The listing builds one solid part. Answer for the finished solid, in the listing's coordinates (mm). Face numbers are marked on the shaded views. A direction names the side the tool comes from. Coordinates: 2 decimals unless noted, no trailing zeros. Loops run counter-clockwise (first coordinate to the right, second up) from the corner with the lowest first, then second, coordinate; pieces in that order, holes last. Notation, with made-up numbers: M 10,2 L 32,2 A27 ccw 32,28 Z; hole C 83,79 d9. An arc over 180 degrees is marked long. Return JSON: item names as keys, results as strings. Group by question number.
1. Which of the six approach directions +Z, -Z, +X, -X, +Y, -Y give full straight-line access (tool end or side, diameter ignored) to the marked faces 1, 2 and 3?
2. Section C-C (y = -13) is taken. Count the separate pieces of the cut face and the enclosed holes in it, then the cut area to 3 significant figures.
3. Section A-A (y = 9.25) is taken. Write down the section's boundary in (x, z), then the cut area to 4 significant figures.
4. Section D-D (y = 3.5) is taken. Write down the section's boundary in (x, z), then the cut area to 3 significant figures.
5. Given P1, Ø4.5, axis at x = 4.5, y = 9.25, coming from the -Z side; P2, Ø8, axis at x = 2.5, y = -20.5, coming from the +Z side; P3, Ø1, axis at x = 2, z = 3, coming from the -Y side; P4, Ø0.6, axis at y = -4.5, z = 0.5, coming from the -X side, each flat-ended and moving along its own axis, determine where each tip first touches the part or whether it passes through.
6. The mould has two halves that part along Y. Classify the marked faces 4, 5 and 6: pulls with the +Y half, pulls with the -Y half, needs draft (parallel to the pull), parting line crosses it, or undercut.
7. Section B-B (y = 17.75) is taken. Write down the section's boundary in (x, z), then the cut area to 4 significant figures.
8. Straight lines are drawn through the part: L1, parallel to Y at x = -11.5, z = 6.75; L2, parallel to X at y = 9.25, z = 1; L3, parallel to X at y = -12, z = 5. For each, find the intervals that lie inside material, in ascending order. Write a range as from..to.
```python
from build123d import *

# Parameters (mm, degrees)
SKETCH_W        = 27.5
SKETCH_H        = 57.5
SKETCH_R        = 1.75
PAD_DEPTH       = 9
POCKET_DEPTH    = 7
SKETCH002_W     = 24.5
SKETCH002_H     = 54.5
POCKET001_DEPTH = 3
SKETCH003_W     = 0.8
SKETCH003_H     = 5
PAD001_DEPTH    = 1.4
CHAMFER_SIZE    = 0.6
SKETCH004_W     = 20
SKETCH004_H     = 3
POCKET002_DEPTH = 9.001
SKETCH005_W     = 22.5
SKETCH005_H     = 2
PAD002_DEPTH    = 2
POCKET003_DEPTH = 2.001
CHAMFER001_SIZE = 2.5


with BuildPart() as part:
    # Sketch → Pad (new body)
    with BuildSketch(Plane.XY):
        Rectangle(SKETCH_W, SKETCH_H)
        with Locations((-4.5, 9.25)):
            Circle(SKETCH_R, mode=Mode.SUBTRACT)
        with Locations((-4.5, -25.75)):
            Circle(SKETCH_R, mode=Mode.SUBTRACT)
        with Locations((4.5, 9.25)):
            Circle(SKETCH_R, mode=Mode.SUBTRACT)
        with Locations((4.5, -25.75)):
            Circle(SKETCH_R, mode=Mode.SUBTRACT)
    extrude(amount=PAD_DEPTH)

    # Sketch001 (on Face10 of Pad) → Pocket (cut)
    with BuildSketch(Plane.XY.offset(9)):
        Polygon((-11.25, 26.25), (11.25, 26.25), (11.25, -26.25), (8, -26.25), (8, -29.25), (-8, -29.25), (-8, -26.25), (-11.25, -26.25), align=None)
    extrude(amount=-POCKET_DEPTH, mode=Mode.SUBTRACT)

    # Sketch002 (on Face5 of Pocket) → Pocket001 (cut)
    with BuildSketch(Plane.XY.offset(9)):
        Rectangle(SKETCH002_W, SKETCH002_H)
    extrude(amount=-POCKET001_DEPTH, mode=Mode.SUBTRACT)

    # Sketch003 (on Face5 of Pocket001) → Pad001 (join)
    with BuildSketch(Plane.XY.offset(9)):
        with Locations((-11.85, 12.5)):
            Rectangle(SKETCH003_W, SKETCH003_H)
        with Locations((-11.85, -12.5)):
            Rectangle(SKETCH003_W, SKETCH003_H)
        with Locations((11.85, -12.5)):
            Rectangle(SKETCH003_W, SKETCH003_H)
        with Locations((11.85, 12.5)):
            Rectangle(SKETCH003_W, SKETCH003_H)
    extrude(amount=-PAD001_DEPTH)

    # Chamfer
    chamfer_edges = [part.edges().sort_by_distance(p)[0] for p in [
        (-11.45, -12.5, 9),
        (-11.45, -12.5, 7.6),
        (-11.45, 12.5, 9),
        (-11.45, 12.5, 7.6),
        (11.45, 12.5, 9),
        (11.45, 12.5, 7.6),
        (11.45, -12.5, 9),
        (11.45, -12.5, 7.6),
    ]]
    chamfer(chamfer_edges, length=CHAMFER_SIZE)

    # Sketch004 (on Face4 of Chamfer) → Pocket002 (cut, through all)
    with BuildSketch(Plane.XY.offset(9)):
        with Locations((0, 27.75)):
            Rectangle(SKETCH004_W, SKETCH004_H)
    extrude(amount=-POCKET002_DEPTH, mode=Mode.SUBTRACT)

    # Sketch005 (on Face22 of Pocket002) → Pad002 (join)
    with BuildSketch(Plane.XY.offset(2)):
        with Locations((0, 25.25)):
            Rectangle(SKETCH005_W, SKETCH005_H)
        with Locations((0, -20)):
            Rectangle(SKETCH005_W, SKETCH005_H)
    extrude(amount=PAD002_DEPTH)

    # Sketch006 (on Face52 of Pad002) → Pocket003 (cut, through all)
    with BuildSketch(Plane.XY.offset(2)):
        with BuildLine():
            ThreePointArc((-7, 21.25), (-10.5, 17.75), (-7, 14.25))
            Line((-7, 14.25), (7, 14.25))
            ThreePointArc((7, 14.25), (10.5, 17.75), (7, 21.25))
            Line((-7, 21.25), (7, 21.25))
        make_face()
        with BuildLine():
            ThreePointArc((-1.5, 1), (-6, 5.5), (-10.5, 1))
            Line((-10.5, 1), (-10.5, -14))
            ThreePointArc((-10.5, -14), (-6, -18.5), (-1.5, -14))
            Line((-1.5, 1), (-1.5, -14))
        make_face()
        with BuildLine():
            ThreePointArc((10.5, 1), (6, 5.5), (1.5, 1))
            Line((1.5, 1), (1.5, -14))
            ThreePointArc((1.5, -14), (6, -18.5), (10.5, -14))
            Line((10.5, 1), (10.5, -14))
        make_face()
    extrude(amount=-POCKET003_DEPTH, mode=Mode.SUBTRACT)

    # Chamfer001
    chamfer001_edges = [part.edges().sort_by_distance(p)[0] for p in [
        (-13.75, 0, 0),
        (13.75, 0, 0),
    ]]
    chamfer(chamfer001_edges, length=CHAMFER001_SIZE)


solid = part.part
```
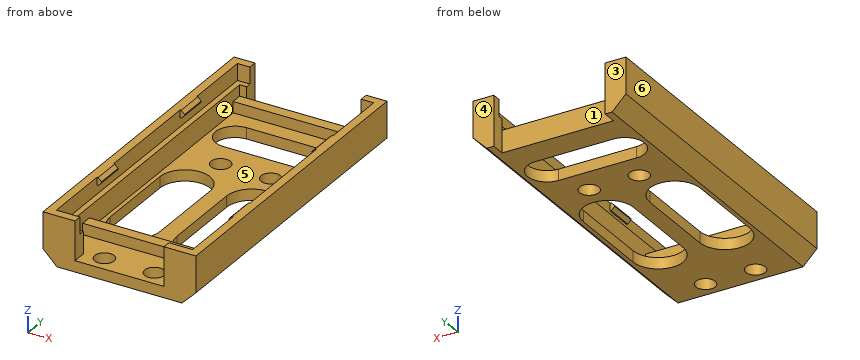
Worked out:
{
 "1": {"face 1": "+Z, -Z, +Y", "face 2": "+Z", "face 3": "+Z, -Z, +X, -X, +Y"},
 "2": {"separate pieces": "3", "enclosed holes": "0", "area": "43.3 mm^2"},
 "3": {"outline": "M -13.75,2.5 L -11.25,0 L -6.25,0 L -6.25,2 L -11.25,2 L -11.25,6 L -12.25,6 L -12.25,9 L -13.75,9 Z; M -2.75,0 L 2.75,0 L 2.75,2 L -2.75,2 Z; M 6.25,0 L 11.25,0 L 13.75,2.5 L 13.75,9 L 12.25,9 L 12.25,6 L 11.25,6 L 11.25,2 L 6.25,2 Z", "area": "63.75 mm^2"},
 "4": {"outline": "M -13.75,2.5 L -11.25,0 L -9.74,0 L -9.74,2 L -11.25,2 L -11.25,6 L -12.25,6 L -12.25,9 L -13.75,9 Z; M -2.26,0 L 2.26,0 L 2.26,2 L -2.26,2 Z; M 9.74,0 L 11.25,0 L 13.75,2.5 L 13.75,9 L 12.25,9 L 12.25,6 L 11.25,6 L 11.25,2 L 9.74,2 Z", "area": "47.8 mm^2"},
 "5": {"P1": "z = 0", "P2": "z = 4", "P3": "y = -21", "P4": "x = -12.05"},
 "6": {"face 4": "pulls with the +Y half", "face 5": "undercut", "face 6": "needs draft"},
 "7": {"outline": "M -13.75,2.5 L -11.25,0 L -10.5,0 L -10.5,2 L -11.25,2 L -11.25,6 L -12.25,6 L -12.25,9 L -13.75,9 Z; M 10.5,0 L 11.25,0 L 13.75,2.5 L 13.75,9 L 12.25,9 L 12.25,6 L 11.25,6 L 11.25,2 L 10.5,2 Z", "area": "35.75 mm^2"},
 "8": {"L1": "-28.75..-27.25, 27.25..28.75", "L2": "-12.25..-6.25, -2.75..2.75, 6.25..12.25", "L3": "-13.75..-11.25, 11.25..13.75"}
}
